Geometry check sheet. Reference: the model listing, model coordinates, mm. Round coordinates to 2 decimals unless told otherwise and drop trailing zeros. Loops run counter-clockwise (first coordinate to the right, second up) from the corner with the lowest first, then second, coordinate; pieces in that order, holes last. Notation, with made-up numbers: (21.5, -4.5) - (33.5, -4.5) arc R34 cw to (33.5, 26.5) - close; hole circle Ø4 at (-10.75, 86). An arc over 180 degrees is marked (long way). Write item = value, one per line.
```python
from build123d import *

# Parameters (mm, degrees)
F0_R     = 3.5
F1_DEPTH = 2
F2_R     = 0.5


with BuildPart() as f1:
    # F0 (on Top) → F1 (new body)
    with BuildSketch(Plane.XY):
        with BuildLine():
            ThreePointArc((38.0882352941, 20.5882352941), (36.6237692001, 24.1237692001), (33.0882352941, 25.5882352941))
            Line((33.0882352941, 25.5882352941), (-31.9117647059, 25.5882352941))
            ThreePointArc((-31.9117647059, 25.5882352941), (-35.4472986118, 24.1237692001), (-36.9117647059, 20.5882352941))
            Line((-36.9117647059, 20.5882352941), (-36.9117647059, -19.4117647059))
            ThreePointArc((-36.9117647059, -19.4117647059), (-35.4472986118, -22.9472986118), (-31.9117647059, -24.4117647059))
            Line((-31.9117647059, -24.4117647059), (33.0882352941, -24.4117647059))
            ThreePointArc((33.0882352941, -24.4117647059), (36.6237692001, -22.9472986118), (38.0882352941, -19.4117647059))
            Line((38.0882352941, -19.4117647059), (38.0882352941, 20.5882352941))
        make_face()
        with BuildLine():
            ThreePointArc((33.0882352941, 24.5882352941), (35.9166624189, 23.4166624189), (37.0882352941, 20.5882352941))
            Line((37.0882352941, 20.5882352941), (37.0882352941, -19.4117647059))
            ThreePointArc((37.0882352941, -19.4117647059), (35.9166624189, -22.2401918306), (33.0882352941, -23.4117647059))
            Line((33.0882352941, -23.4117647059), (-31.9117647059, -23.4117647059))
            ThreePointArc((-31.9117647059, -23.4117647059), (-34.7401918306, -22.2401918306), (-35.9117647059, -19.4117647059))
            Line((-35.9117647059, -19.4117647059), (-35.9117647059, 20.5882352941))
            ThreePointArc((-35.9117647059, 20.5882352941), (-34.7401918306, 23.4166624189), (-31.9117647059, 24.5882352941))
            Line((-31.9117647059, 24.5882352941), (33.0882352941, 24.5882352941))
        make_face(mode=Mode.SUBTRACT)
        with BuildLine():
            Line((37.0882352941, -19.4117647059), (37.0882352941, 20.5882352941))
            ThreePointArc((37.0882352941, 20.5882352941), (35.9166624189, 23.4166624189), (33.0882352941, 24.5882352941))
            Line((33.0882352941, 24.5882352941), (-31.9117647059, 24.5882352941))
            ThreePointArc((-31.9117647059, 24.5882352941), (-34.7401918306, 23.4166624189), (-35.9117647059, 20.5882352941))
            Line((-35.9117647059, 20.5882352941), (-35.9117647059, -19.4117647059))
            ThreePointArc((-35.9117647059, -19.4117647059), (-34.7401918306, -22.2401918306), (-31.9117647059, -23.4117647059))
            Line((-31.9117647059, -23.4117647059), (33.0882352941, -23.4117647059))
            ThreePointArc((33.0882352941, -23.4117647059), (35.9166624189, -22.2401918306), (37.0882352941, -19.4117647059))
        make_face()
        with BuildLine():
            ThreePointArc((33.0882352941, 23.0882352941), (34.8560022471, 22.3560022471), (35.5882352941, 20.5882352941))
            Line((35.5882352941, 20.5882352941), (35.5882352941, -19.4117647059))
            ThreePointArc((35.5882352941, -19.4117647059), (34.8560022471, -21.1795316588), (33.0882352941, -21.9117647059))
            Line((33.0882352941, -21.9117647059), (-31.9117647059, -21.9117647059))
            ThreePointArc((-31.9117647059, -21.9117647059), (-33.6795316588, -21.1795316588), (-34.4117647059, -19.4117647059))
            Line((-34.4117647059, -19.4117647059), (-34.4117647059, 20.5882352941))
            ThreePointArc((-34.4117647059, 20.5882352941), (-33.6795316588, 22.3560022471), (-31.9117647059, 23.0882352941))
            Line((-31.9117647059, 23.0882352941), (33.0882352941, 23.0882352941))
        make_face(mode=Mode.SUBTRACT)
        with BuildLine():
            Line((35.5882352941, -19.4117647059), (35.5882352941, 20.5882352941))
            ThreePointArc((35.5882352941, 20.5882352941), (34.8560022471, 22.3560022471), (33.0882352941, 23.0882352941))
            Line((33.0882352941, 23.0882352941), (-31.9117647059, 23.0882352941))
            ThreePointArc((-31.9117647059, 23.0882352941), (-33.6795316588, 22.3560022471), (-34.4117647059, 20.5882352941))
            Line((-34.4117647059, 20.5882352941), (-34.4117647059, -19.4117647059))
            ThreePointArc((-34.4117647059, -19.4117647059), (-33.6795316588, -21.1795316588), (-31.9117647059, -21.9117647059))
            Line((-31.9117647059, -21.9117647059), (33.0882352941, -21.9117647059))
            ThreePointArc((33.0882352941, -21.9117647059), (34.8560022471, -21.1795316588), (35.5882352941, -19.4117647059))
        make_face()
        with BuildLine():
            ThreePointArc((33.0882352941, 22.0882352941), (34.1488954659, 21.6488954659), (34.5882352941, 20.5882352941))
            Line((34.5882352941, 20.5882352941), (34.5882352941, 14.3133180765))
            Line((34.5882352941, 14.3133180765), (34.5882352941, -13.1368474882))
            Line((34.5882352941, -13.1368474882), (34.5882352941, -19.4117647059))
            ThreePointArc((34.5882352941, -19.4117647059), (34.1488954659, -20.4724248777), (33.0882352941, -20.9117647059))
            Line((33.0882352941, -20.9117647059), (26.8133180765, -20.9117647059))
            Line((26.8133180765, -20.9117647059), (-25.6368474882, -20.9117647059))
            Line((-25.6368474882, -20.9117647059), (-31.9117647059, -20.9117647059))
            ThreePointArc((-31.9117647059, -20.9117647059), (-32.9724248777, -20.4724248777), (-33.4117647059, -19.4117647059))
            Line((-33.4117647059, -19.4117647059), (-33.4117647059, -13.1368474882))
            Line((-33.4117647059, -13.1368474882), (-33.4117647059, 14.3133180765))
            Line((-33.4117647059, 14.3133180765), (-33.4117647059, 20.5882352941))
            ThreePointArc((-33.4117647059, 20.5882352941), (-32.9724248777, 21.6488954659), (-31.9117647059, 22.0882352941))
            Line((-31.9117647059, 22.0882352941), (-25.6368474882, 22.0882352941))
            Line((-25.6368474882, 22.0882352941), (26.8133180765, 22.0882352941))
            Line((26.8133180765, 22.0882352941), (33.0882352941, 22.0882352941))
        make_face(mode=Mode.SUBTRACT)
        with BuildLine():
            Line((34.5882352941, -13.1368474882), (34.5882352941, 14.3133180765))
            ThreePointArc((34.5882352941, 14.3133180765), (26.6991479976, 14.1991479976), (26.8133180765, 22.0882352941))
            Line((26.8133180765, 22.0882352941), (-25.6368474882, 22.0882352941))
            ThreePointArc((-25.6368474882, 22.0882352941), (-25.5226774094, 14.1991479976), (-33.4117647059, 14.3133180765))
            Line((-33.4117647059, 14.3133180765), (-33.4117647059, -13.1368474882))
            ThreePointArc((-33.4117647059, -13.1368474882), (-25.5226774094, -13.0226774094), (-25.6368474882, -20.9117647059))
            Line((-25.6368474882, -20.9117647059), (26.8133180765, -20.9117647059))
            ThreePointArc((26.8133180765, -20.9117647059), (26.6991479976, -13.0226774094), (34.5882352941, -13.1368474882))
        make_face()
        with BuildLine():
            ThreePointArc((-33.4117647059, 14.3133180765), (-25.5226774094, 14.1991479976), (-25.6368474882, 22.0882352941))
            Line((-25.6368474882, 22.0882352941), (-31.9117647059, 22.0882352941))
            ThreePointArc((-31.9117647059, 22.0882352941), (-32.9724248777, 21.6488954659), (-33.4117647059, 20.5882352941))
            Line((-33.4117647059, 20.5882352941), (-33.4117647059, 14.3133180765))
        make_face()
        with Locations((-29.4117647059, 18.0882352941)):
            Circle(F0_R, mode=Mode.SUBTRACT)
        with BuildLine():
            Line((-31.9117647059, -20.9117647059), (-25.6368474882, -20.9117647059))
            ThreePointArc((-25.6368474882, -20.9117647059), (-25.5226774094, -13.0226774094), (-33.4117647059, -13.1368474882))
            Line((-33.4117647059, -13.1368474882), (-33.4117647059, -19.4117647059))
            ThreePointArc((-33.4117647059, -19.4117647059), (-32.9724248777, -20.4724248777), (-31.9117647059, -20.9117647059))
        make_face()
        with Locations((-29.4117647059, -16.9117647059)):
            Circle(F0_R, mode=Mode.SUBTRACT)
        with BuildLine():
            Line((34.5882352941, 14.3133180765), (34.5882352941, 20.5882352941))
            ThreePointArc((34.5882352941, 20.5882352941), (34.1488954659, 21.6488954659), (33.0882352941, 22.0882352941))
            Line((33.0882352941, 22.0882352941), (26.8133180765, 22.0882352941))
            ThreePointArc((26.8133180765, 22.0882352941), (26.6991479976, 14.1991479976), (34.5882352941, 14.3133180765))
        make_face()
        with Locations((30.5882352941, 18.0882352941)):
            Circle(F0_R, mode=Mode.SUBTRACT)
        with BuildLine():
            Line((34.5882352941, -19.4117647059), (34.5882352941, -13.1368474882))
            ThreePointArc((34.5882352941, -13.1368474882), (26.6991479976, -13.0226774094), (26.8133180765, -20.9117647059))
            Line((26.8133180765, -20.9117647059), (33.0882352941, -20.9117647059))
            ThreePointArc((33.0882352941, -20.9117647059), (34.1488954659, -20.4724248777), (34.5882352941, -19.4117647059))
        make_face()
        with Locations((30.5882352941, -16.9117647059)):
            Circle(F0_R, mode=Mode.SUBTRACT)
    extrude(amount=F1_DEPTH)

    # F2
    f2_edges = [f1.edges().sort_by_distance(p)[0] for p in [
        (-36.911765, 0.588235, 2),
    ]]
    fillet(f2_edges, radius=F2_R)


solid = f1.part
```
(1) Scan lines: L1, parallel to X at y = -17.5, z = 1.3; L2, parallel to Y at x = 31.5, z = 0.65; L3, parallel to Y at x = -30, z = 1.35. Record each from-to range of solid material in increasing order. Write a range as [from, to].
Answers follow:
L1 = [-36.91, -32.86], [-25.96, 27.14], [34.04, 38.09]
L2 = [-24.41, -20.29], [-13.53, 14.71], [21.47, 25.59]
L3 = [-24.41, -20.36], [-13.46, 14.64], [21.54, 25.59]
(2) Section check A-A (x = -30.5). Enter the section's corners in (y, z), then the cut area to 3 significant figures.
Answers follow:
outline = (-24.41, 0) - (-20.24, 0) - (-20.24, 2) - (-23.91, 2) arc R0.5 ccw to (-24.41, 1.5) - close; (-13.59, 0) - (14.76, 0) - (14.76, 2) - (-13.59, 2) - close; (21.41, 0) - (25.59, 0) - (25.59, 1.5) arc R0.5 ccw to (25.09, 2) - (21.41, 2) - close
area = 73.3 mm²
(3) Mould release check, pull along Y, two halves, no side actions. Record for faces 1 (the flat face through (0, 1, 0)), 2 (the cylindrical face through (33.8, 16.7, 1)), 3 (the flat face through (0, -24.412, 1)): pulls with the +Y half, pulls with the -Y half, needs draft (parallel to the pull), parting line crosses it, or undercut.
Answers follow:
face_1 = needs draft
face_2 = undercut
face_3 = pulls with the -Y half
(4) Section check B-B (y = 16). Enter the section's corners in (x, z), then the cut area to 3 significant figures.
Answers follow:
outline = (-36.91, 0) - (-32.22, 0) - (-32.22, 2) - (-36.41, 2) arc R0.5 ccw to (-36.91, 1.5) - close; (-26.6, 0) - (27.78, 0) - (27.78, 2) - (-26.6, 2) - close; (33.4, 0) - (38.09, 0) - (38.09, 1.5) arc R0.5 ccw to (37.59, 2) - (33.4, 2) - close
area = 127 mm²
(5) Gauge pin test, flat end, axial feed: pin 1 (9 mm diameter, centred on x = -29.41, y = -16.91, fed in from +Z). Record the tip position at first contact, or that the pin passes through.
Answers follow:
pin_1 = 2
(6) Section check C-C (z = 0.9). Enter the section's corners in (x, y).
Answers follow:
outline = (-36.91, -19.41) arc R5 ccw to (-31.91, -24.41) - (33.09, -24.41) arc R5 ccw to (38.09, -19.41) - (38.09, 20.59) arc R5 ccw to (33.09, 25.59) - (-31.91, 25.59) arc R5 ccw to (-36.91, 20.59) - close; hole circle Ø7 at (-29.41, -16.91); hole circle Ø7 at (-29.41, 18.09); hole circle Ø7 at (30.59, -16.91); hole circle Ø7 at (30.59, 18.09)
